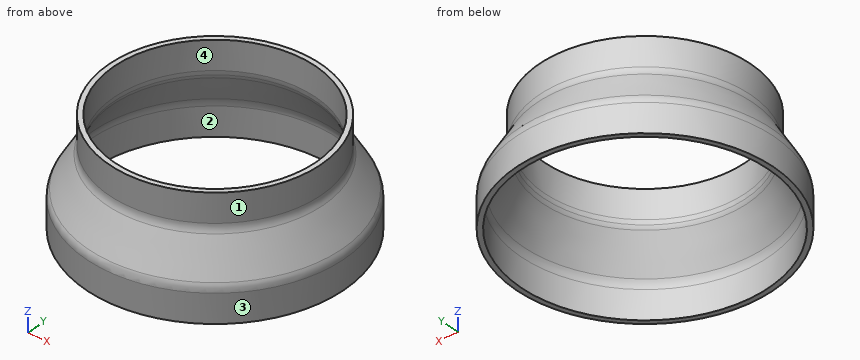
```python
from build123d import *


with BuildPart() as f1:
    # F0 (on Front) → F1 (revolve)
    with BuildSketch(Plane.XZ):
        with BuildLine():
            ThreePointArc((61.36567, 10.486363), (61.779417, 9.295344), (62.339746, 8.165855))
            Line((62.339746, 8.165855), (73.660254, -11.44184))
            ThreePointArc((73.660254, -11.44184), (74.659258, -13.853649), (75, -16.44184))
            Line((75, -16.44184), (75, -33.762348))
            Line((75, -33.762348), (78, -33.762348))
            Line((78, -33.762348), (78, -16.44184))
            ThreePointArc((78, -16.44184), (77.659258, -13.853649), (76.660254, -11.44184))
            Line((76.660254, -11.44184), (65.339746, 8.165855))
            ThreePointArc((65.339746, 8.165855), (64.340742, 10.577665), (64, 13.165855))
            Line((64, 13.165855), (64, 30.486363))
            Line((64, 30.486363), (61, 30.486363))
            Line((61, 30.486363), (61, 13.165855))
            ThreePointArc((61, 13.165855), (61.091839, 11.813691), (61.36567, 10.486363))
        make_face()
    revolve(axis=Axis((0, 0, 3.03654), (0, 0, 1)))


solid = f1.part
```
Source: CAD feature listing. Evaluate the final solid. Frame: model axes, mm. Face numbers are marked on the shaded views. A direction names the side the tool comes from. Round coordinates to 2 decimals unless told otherwise and drop trailing zeros. Loops run counter-clockwise (first coordinate to the right, second up) from the corner with the lowest first, then second, coordinate; pieces in that order, holes last.
(1) Section query D-D (z = 1). Output: boundary loops of the cut face in (x, y), and give its area (3 significant figures).
From the geometry:
outline: circle Ø138.95 at (0, 0); hole circle Ø132.95 at (0, 0)
area: 1,280 mm2
(2) Access query for the marked faces 1 and 2. Directions: +Z, -Z, +X, -X, +Y, -Y. A direction counts if a zero-diameter tool reaches every point of the face in a straight line with its end or side. Return the directions, or none.
From the geometry:
face 1: +Z
face 2: -Z
(3) Contact query for flat-ended pins moving along their axis: pin 1 Ø2 at (x, z) = (-7.5, -23.5) entering from -Y; pin 2 Ø1 at (x, z) = (4.5, -2.5) entering from -Y; pin 3 Ø1.5 at (x, z) = (11.5, 14.5) entering from +Y. Output: stop coordinate, or through.
From the geometry:
pin 1: stops at y = -77.73
pin 2: stops at y = -71.65
pin 3: stops at y = 63.09
(4) Material intervals for probe 1 along Y at (x, z) = (0, -27); probe 2 along Y at (x, z) = (0, 26.5); probe 3 along X at (y, z) = (-40, 3.5), sorted ascending.
From the geometry:
probe 1: y = -78 to -75, 75 to 78
probe 2: y = -64 to -61, 61 to 64
probe 3: x = -55.03 to -51.28, 51.28 to 55.03
(5) Section query A-A (y = 0). Output: boundary loops of the cut face in (x, z).
From the geometry:
outline: (-78, -33.76) - (-75, -33.76) - (-75, -16.44) arc R10 cw to (-73.66, -11.44) - (-62.34, 8.17) arc R10 ccw to (-61.37, 10.49) arc R10 ccw to (-61, 13.17) - (-61, 30.49) - (-64, 30.49) - (-64, 13.17) arc R10 cw to (-65.34, 8.17) - (-76.66, -11.44) arc R10 ccw to (-78, -16.44) - close; (61, 13.17) arc R10 ccw to (61.37, 10.49) arc R10 ccw to (62.34, 8.17) - (73.66, -11.44) arc R10 cw to (75, -16.44) - (75, -33.76) - (78, -33.76) - (78, -16.44) arc R10 ccw to (76.66, -11.44) - (65.34, 8.17) arc R10 cw to (64, 13.17) - (64, 30.49) - (61, 30.49) - close
(6) Section query C-C (z = -24). Output: boundary loops of the cut face in (x, y), and give its area (3 significant figures).
From the geometry:
outline: circle Ø156 at (0, 0); hole circle Ø150 at (0, 0)
area: 1,440 mm2
(7) Pull-direction query (X, two-part tool) for the marked faces 3 and 4; classes: +X half, -X half, draft (parallel to the pull), parting line (faces both ways), or undercut.
From the geometry:
face 3: parting line
face 4: undercut
